Could you check a few things on this model? Use its own coordinates, in mm. A direction names the side the tool comes from. Give positions to 0.01 mm unless a question says otherwise; leave off trailing zeros. Loops run counter-clockwise (first coordinate to the right, second up) from the corner with the lowest first, then second, coordinate; pieces in that order, holes last. Notation, with made-up numbers: (-35, -36) -> (7, -36) arc R34 ccw to (7, 0) -> close; hole circle Ø5 at (27.25, -21). An arc over 180 degrees is marked (long way). Put each result on its own line as item: value.
```python
from build123d import *

# Parameters (mm, degrees)
F1_DEPTH = 5
F0_R     = 7
F2_DEPTH = 5
F3_R     = 15
F3_R_2   = 10
F4_DEPTH = 18
F5_W     = 9.2795909345
F5_H     = 53.3426658501
F6_DEPTH = 18
F7_R     = 1.65
F8_DEPTH = 11.3


with BuildPart() as f1:
    # F0 (on Top) → F1 (new body)
    with BuildSketch(Plane.XY):
        with BuildLine():
            Line((-29, -16.7705098312), (-29, -22.1641602593))
            ThreePointArc((-29, -22.1641602593), (36.5, 0), (-29, 22.1641602593))
            Line((-29, 22.1641602593), (-29, 16.7705098312))
            ThreePointArc((-29, 16.7705098312), (33.5, 0), (-29, -16.7705098312))
        make_face()
    extrude(amount=F1_DEPTH)

    # F0 (on Top) → F2 (join)
    with BuildSketch(Plane.XY):
        with BuildLine():
            Line((-29, -22.1641602593), (-29, -26.6713329251))
            ThreePointArc((-29, -26.6713329251), (39.4, 0), (-29, 26.6713329251))
            Line((-29, 26.6713329251), (-29, 22.1641602593))
            ThreePointArc((-29, 22.1641602593), (36.5, 0), (-29, -22.1641602593))
        make_face()
        with BuildLine():
            Line((-29, -16.7705098312), (-29, -22.1641602593))
            ThreePointArc((-29, -22.1641602593), (36.5, 0), (-29, 22.1641602593))
            Line((-29, 22.1641602593), (-29, 16.7705098312))
            ThreePointArc((-29, 16.7705098312), (33.5, 0), (-29, -16.7705098312))
        make_face()
        with BuildLine():
            Line((-29, 16.7705098312), (-29, -16.7705098312))
            ThreePointArc((-29, -16.7705098312), (33.5, 0), (-29, 16.7705098312))
        make_face()
        Circle(F0_R, mode=Mode.SUBTRACT)
    extrude(amount=-F2_DEPTH)

    # F3 (on face) → F4 (join)
    with BuildSketch(Plane(origin=(0, 0, -5), x_dir=(1, 0, 0), z_dir=(0, 0, -1))):
        Circle(F3_R)
        Circle(F3_R_2, mode=Mode.SUBTRACT)
    extrude(amount=F4_DEPTH)

    # F5 (on face) → F6 (join)
    with BuildSketch(Plane(origin=(0, 0, -5), x_dir=(1, 0, 0), z_dir=(0, 0, -1))):
        with Locations((-24.3602045327, 0)):
            Rectangle(F5_W, F5_H)
    extrude(amount=F6_DEPTH)

    # F7 (on face) → F8 (cut)
    with BuildSketch(Plane(origin=(-29, 0, 0), x_dir=(0, -1, 0), z_dir=(-1, 0, 0))):
        with Locations((-18, -13)):
            Circle(F7_R)
        with Locations((0, -13)):
            Circle(F7_R)
        with Locations((18, -13)):
            Circle(F7_R)
    extrude(amount=-F8_DEPTH, mode=Mode.SUBTRACT)


solid = f1.part
```
1. For faces 1 (the face through (-2.17, 9.76, -13.87)), 2 (the face through (-19.72, 0, -16)), 3 (the face through (36.478, -1.272, 2.465)), 4 (the face through (-24.4, 0.4, -14.6)), which set-ups out of +Z, -Z, +X, -X, +Y, -Y let a thin tool reach every point of the face, with its end or its side?
Recorded:
face 1: -Z
face 2: -Z, +Y, -Y
face 3: +Z
face 4: -X
2. Thinking about a two-plate mould opening in X: for faces 5 (the face through (6.466, -2.681, -2.465)), 6 (the face through (-24, -26.671, -14)), 7 (the face through (-29, 0, -9)), which applies, pulls with the +X half, pulls with the -X half, needs draft (parallel to the pull), parting line crosses it, or undercut?
Recorded:
face 5: undercut
face 6: needs draft
face 7: pulls with the -X half
3. If we section it at D-D (y = -18): List the corners of the cut face in (x, z) for me, then the cut area to 3 significant figures.
Recorded:
outline: (-29, -23) -> (-19.72, -23) -> (-19.72, -14.65) -> (-29, -14.65) -> close; (-29, -11.35) -> (-19.72, -11.35) -> (-19.72, -5) -> (35.05, -5) -> (35.05, 0) -> (31.75, 0) -> (31.75, 5) -> (28.25, 5) -> (28.25, 0) -> (-28.25, 0) -> (-28.25, 5) -> (-29, 5) -> close
area: 478 mm^2
4. If we section it at B-B (y = 0): List the corners of the cut face in (x, z) for me.
Recorded:
outline: (-29, -23) -> (-19.72, -23) -> (-19.72, -14.65) -> (-29, -14.65) -> close; (-29, -11.35) -> (-19.72, -11.35) -> (-19.72, -5) -> (-15, -5) -> (-15, -23) -> (-10, -23) -> (-10, -5) -> (-7, -5) -> (-7, 0) -> (-29, 0) -> close; (7, -5) -> (10, -5) -> (10, -23) -> (15, -23) -> (15, -5) -> (39.4, -5) -> (39.4, 0) -> (36.5, 0) -> (36.5, 5) -> (33.5, 5) -> (33.5, 0) -> (7, 0) -> close
5. If we section it at A-A (x = 0): List the corners of the cut face in (y, z) for me, then the cut area to 3 significant figures.
Recorded:
outline: (-39.4, -5) -> (-15, -5) -> (-15, -23) -> (-10, -23) -> (-10, -5) -> (-7, -5) -> (-7, 0) -> (-33.5, 0) -> (-33.5, 5) -> (-36.5, 5) -> (-36.5, 0) -> (-39.4, 0) -> close; (7, -5) -> (10, -5) -> (10, -23) -> (15, -23) -> (15, -5) -> (39.4, -5) -> (39.4, 0) -> (36.5, 0) -> (36.5, 5) -> (33.5, 5) -> (33.5, 0) -> (7, 0) -> close
area: 534 mm^2
6. I'm going to push flat-ended pins straight in: pin 1 (16 mm diameter, centred on x = 0, y = 0, fed in from -Z); pin 2 (6 mm diameter, centred on x = 10.5, y = -17, fed in from +Z); pin 3 (10 mm diameter, centred on x = -7.5, z = -4, fed in from +Y); pin 4 (3 mm diameter, centred on y = -18, z = -13, fed in from -X). Where does each tip first touch, or does it pass through?
Recorded:
pin 1: stops at z = -5
pin 2: stops at z = 0
pin 3: stops at y = 39.32
pin 4: passes through
7. If we section it at C-C (x = -21): List the corners of the cut face in (y, z) for me, then the cut area to 3 significant figures.
Recorded:
outline: (-33.34, -5) -> (-26.67, -5) -> (-26.67, -23) -> (26.67, -23) -> (26.67, -5) -> (33.34, -5) -> (33.34, 0) -> (29.85, 0) -> (29.85, 5) -> (26.1, 5) -> (26.1, 0) -> (-26.1, 0) -> (-26.1, 5) -> (-29.85, 5) -> (-29.85, 0) -> (-33.34, 0) -> close; hole circle Ø3.3 at (-18, -13); hole circle Ø3.3 at (0, -13); hole circle Ø3.3 at (18, -13)
area: 1,310 mm^2
8. I need wall thicknesses on line 1 (X direction, y = -3.5, z = -14.25); line 2 (Y direction, x = 0, z = 3.9); line 3 (Z direction, x = -27, y = 18). Which ranges of each line are inside material? Lowest first, please.
Recorded:
line 1: x = -29 to -19.72, -14.59 to -9.37, 9.37 to 14.59
line 2: y = -36.5 to -33.5, 33.5 to 36.5
line 3: z = -23 to -14.65, -11.35 to 0
